Input: part model. Units: mm. Frame: model coordinates. Round coordinates to 2 decimals unless told otherwise and drop trailing zeros. Loops run counter-clockwise (first coordinate to the right, second up) from the corner with the lowest first, then second, coordinate; pieces in that order, holes last.
(1) Cut plane A-A, the plane y = 0. Output: boundary loops of the cut face in (x, z) (3 decimals), and give its area (3 significant figures).
(2) Cut plane C-C, the plane x = 50. Output: boundary loops of the cut face in (y, z) (3 decimals).
(3) Line query: line 1 (Y direction, x = 0, z = 2.1) (3 decimals); line 2 (Y direction, x = 50, z = 1.2) (3 decimals); line 3 (Y direction, x = 1, z = 2.15) (3 decimals). Output: solid intervals per line, ascending.
(4) Draft query along Y for faces 1 (the face through (-1, 63.175, 2)), 2 (the face through (51.35, 28.97, 1.57)), 3 (the face through (-63.175, -1, 2)), 4 (the face through (-48.65, -31.03, 1.57)). Return one class per face: released by +Y, released by -Y, zero draft, split by the parting line, or undercut.
from build123d import *

# Parameters (mm, degrees)
SKETCH1_W           = 126.35
SKETCH1_H           = 126.35
BOSS_EXTRUDE1_DEPTH = 3.175
SKETCH2_R           = 1.7
CUT_EXTRUDE1_DEPTH  = 7


with BuildPart() as part:
    # Sketch1 → Boss-Extrude1 (new body)
    with BuildSketch(Plane.XY):
        Rectangle(SKETCH1_W, SKETCH1_H)
    extrude(amount=BOSS_EXTRUDE1_DEPTH)

    # Sketch2 → Cut-Extrude1 (cut)
    with BuildSketch(Plane(origin=(-17.047760395, -31.681970197, 0), x_dir=(-1, 0, 0), z_dir=(0, 0, -1))):
        with Locations((-17.047760395, -18.318029803)):
            Circle(SKETCH2_R)
        with Locations((12.952239605, -18.318029803)):
            Circle(SKETCH2_R)
        with Locations((-47.047760395, -18.318029803)):
            Circle(SKETCH2_R)
        with Locations((-67.047760395, 61.681970197)):
            Circle(SKETCH2_R)
        with Locations((-67.047760395, 31.681970197)):
            Circle(SKETCH2_R)
        with Locations((-67.047760395, 1.681970197)):
            Circle(SKETCH2_R)
        with Locations((12.952239605, 81.681970197)):
            Circle(SKETCH2_R)
        with Locations((-17.047760395, 81.681970197)):
            Circle(SKETCH2_R)
        with Locations((-47.047760395, 81.681970197)):
            Circle(SKETCH2_R)
        with Locations((32.952239605, 1.681970197)):
            Circle(SKETCH2_R)
        with Locations((32.952239605, 31.681970197)):
            Circle(SKETCH2_R)
        with Locations((32.952239605, 61.681970197)):
            Circle(SKETCH2_R)
    extrude(amount=-CUT_EXTRUDE1_DEPTH, mode=Mode.SUBTRACT)


solid = part.part
Reported:
1. outline: (-63.175, 0) - (-51.7, 0) - (-51.7, 3.175) - (-63.175, 3.175) - close; (-48.3, 0) - (48.3, 0) - (48.3, 3.175) - (-48.3, 3.175) - close; (51.7, 0) - (63.175, 0) - (63.175, 3.175) - (51.7, 3.175) - close
1. area: 380 mm2
2. outline: (-63.175, 0) - (-31.7, 0) - (-31.7, 3.175) - (-63.175, 3.175) - close; (-28.3, 0) - (-1.7, 0) - (-1.7, 3.175) - (-28.3, 3.175) - close; (1.7, 0) - (28.3, 0) - (28.3, 3.175) - (1.7, 3.175) - close; (31.7, 0) - (63.175, 0) - (63.175, 3.175) - (31.7, 3.175) - close
3. line 1: y = -63.175 to -51.7, -48.3 to 48.3, 51.7 to 63.175
3. line 2: y = -63.175 to -31.7, -28.3 to -1.7, 1.7 to 28.3, 31.7 to 63.175
3. line 3: y = -63.175 to -51.375, -48.625 to 48.625, 51.375 to 63.175
4. face 1: released by +Y
4. face 2: undercut
4. face 3: zero draft
4. face 4: undercut
